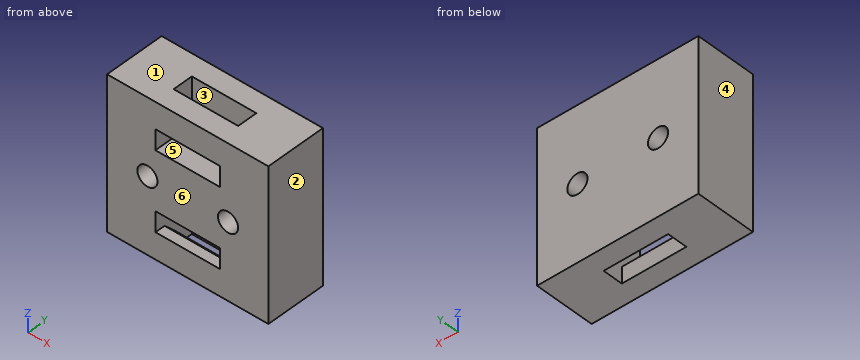
from build123d import *

# Parameters (mm, degrees)
CROQUIS1_W              = 16
CROQUIS1_H              = 15
CROQUIS1_R              = 1
SALIENTE_EXTRUIR1_DEPTH = 6
CROQUIS6_W              = 6.4
CROQUIS6_H              = 2
CORTAR_EXTRUIR3_DEPTH   = 32
CROQUIS7_W              = 6.4
CROQUIS7_H              = 2
CORTAR_EXTRUIR4_DEPTH   = 4.6
CROQUIS8_W              = 6.4
CROQUIS8_H              = 2
SALIENTE_EXTRUIR5_DEPTH = 2
CHAFL_N1_SIZE           = 1


with BuildPart() as part:
    # Croquis1 → Saliente-Extruir1 (new body)
    with BuildSketch(Plane(origin=(0, 0, 0), x_dir=(1, 0, 0), z_dir=(0, 1, 0))):
        Rectangle(CROQUIS1_W, CROQUIS1_H)
        with Locations((4, 0)):
            Circle(CROQUIS1_R, mode=Mode.SUBTRACT)
        with Locations((-4, 0)):
            Circle(CROQUIS1_R, mode=Mode.SUBTRACT)
    extrude(amount=SALIENTE_EXTRUIR1_DEPTH)

    # Croquis6 → Cortar-Extruir3 (cut)
    with BuildSketch(Plane(origin=(0, 6, 0), x_dir=(1, 0, 0), z_dir=(0, 1, 0))):
        with Locations((0, -3.9)):
            Rectangle(CROQUIS6_W, CROQUIS6_H)
        with Locations((0, 3.9)):
            Rectangle(CROQUIS6_W, CROQUIS6_H)
    cortar_extruir3 = extrude(amount=-CORTAR_EXTRUIR3_DEPTH, mode=Mode.SUBTRACT)

    # Croquis7 → Cortar-Extruir4 (cut)
    with BuildSketch(Plane(origin=(0, 0, 7.5), x_dir=(-1, 0, 0), z_dir=(0, 0, -1))):
        with Locations((0, 3)):
            Rectangle(CROQUIS7_W, CROQUIS7_H)
    cortar_extruir4 = extrude(amount=CORTAR_EXTRUIR4_DEPTH, mode=Mode.SUBTRACT)

    # Simetría1: Cortar-Extruir3, Cortar-Extruir4 across plane
    add(cortar_extruir3.mirror(Plane.XY), mode=Mode.SUBTRACT)
    add(cortar_extruir4.mirror(Plane.XY), mode=Mode.SUBTRACT)

    # Croquis8 → Saliente-Extruir5 (add)
    with BuildSketch(Plane(origin=(0, 6, 0), x_dir=(1, 0, 0), z_dir=(0, 1, 0))):
        with Locations((0, 3.9)):
            Rectangle(CROQUIS8_W, CROQUIS8_H)
        with Locations((0, -3.9)):
            Rectangle(CROQUIS8_W, CROQUIS8_H)
    extrude(amount=-SALIENTE_EXTRUIR5_DEPTH)

    # Chaflán1
    chafl_n1_edges = [part.edges().sort_by_distance(p)[0] for p in [
        (0, 2, -4.9),
        (0, 2, 4.9),
    ]]
    chamfer(chafl_n1_edges, length=CHAFL_N1_SIZE)


solid = part.part
The model under review builds one solid part; all positions refer to its coordinate system, in mm. Face numbers are marked on the shaded views. A direction names the side the tool comes from. Round coordinates to 2 decimals unless told otherwise and drop trailing zeros. Loops run counter-clockwise (first coordinate to the right, second up) from the corner with the lowest first, then second, coordinate; pieces in that order, holes last. Notation, with made-up numbers: M 35.25,-17.75 L 88.25,-17.75 A23 ccw 88.25,9.25 Z; hole C 42.25,-32.75 d11. An arc over 180 degrees is marked long. Answer as CSV lines item,"result".
1. We need section D-D (y = 4.8). Give the boundary of the cut face in (x, z), plus the area to 3 significant figures.
Outcome:
outline,"M -8,-7.5 L 8,-7.5 L 8,7.5 L -8,7.5 Z; hole C -4,0 d2; hole C 4,0 d2"
area,"234 mm2"
2. Insertion check: pin 1 Ø1.5 at (x, z) = (4, 2) entering from -Y. The pin has a flat end and moves straight along its axis. Give the tip position at first contact, or say it passes through.
Outcome:
pin 1,"stops at y = 0"
3. To check wall thickness, follow L1, parallel to X at y = 3.5, z = 0; L2, parallel to Z at x = 4, y = 4.9; L3, parallel to X at y = 0.9, z = -0.5. State the ranges of each line that lie inside material, in increasing order. Write a range as [from, to].
Outcome:
L1,"x = [-8, -5], [-3, 3], [5, 8]"
L2,"z = [-7.5, -1], [1, 7.5]"
L3,"x = [-8, -4.87], [-3.13, 3.13], [4.87, 8]"
4. Draft analysis for pull direction X (two halves, no side actions). For the marked faces 1, 2, 3 and 4, state which applies: pulls with the +X half, pulls with the -X half, needs draft (parallel to the pull), parting line crosses it, or undercut.
Outcome:
face 1,"needs draft"
face 2,"pulls with the +X half"
face 3,"undercut"
face 4,"pulls with the -X half"
5. We need section B-B (x = 4). Give the boundary of the cut face in (y, z), plus the area to 3 significant figures.
Outcome:
outline,"M 0,-7.5 L 6,-7.5 L 6,-1 L 0,-1 Z; M 0,1 L 6,1 L 6,7.5 L 0,7.5 Z"
area,"78.0 mm2"
6. We need section A-A (z = 0). Give the boundary of the cut face in (x, y).
Outcome:
outline,"M -8,0 L -5,0 L -5,6 L -8,6 Z; M -3,0 L 3,0 L 3,6 L -3,6 Z; M 5,0 L 8,0 L 8,6 L 5,6 Z"
7. We need section C-C (x = -1.5). Give the boundary of the cut face in (y, z).
Outcome:
outline,"M 0,-7.5 L 2,-7.5 L 2,-5.9 L 1,-4.9 L 0,-4.9 Z; M 0,-2.9 L 4,-2.9 L 4,-7.5 L 6,-7.5 L 6,7.5 L 4,7.5 L 4,2.9 L 0,2.9 Z; M 0,4.9 L 1,4.9 L 2,5.9 L 2,7.5 L 0,7.5 Z"
8. For the marked faces 5 and 6, list the 3-axis set-ups (+Z, -Z, +X, -X, +Y, -Y) from which the entire face can be reached by the end or side of a thin tool; tool diameter is ignored.
Outcome:
face 5,"-Y"
face 6,"+Z, -Z, +X, -X, -Y"
